Could you check a few things on this model? Use its own coordinates, in mm. A direction names the side the tool comes from. Coordinates: 2 decimals unless noted, no trailing zeros. Write each loop counter-clockwise with the first axis right and the second up, starting at its lowest first coordinate (ties: lowest second). Pieces come first, ordered by that corner, then holes.
Item 1: If I drill on probe 1 along Z at (x, y) = (-2.75, -4); probe 2 along X at (y, z) = (-1.25, 2.05); probe 3 along X at (y, z) = (5, 0.7), over which ranges is the centre line in solid material (lowest first)?
Item 2: I want a section at B-B on z = 2.8. Please give me the cut outline in (x, y), then the cut area to 3 significant figures.
Item 3: I want a section at A-A on z = 2. Please give me the cut outline in (x, y), then the cut area to 3 significant figures.
Item 4: For P1, Ø1, axis at x = -3.5, y = 5, coming from the +Z side, with a flat end and sliding along its axis, tell me the tip position at first contact or that it passes through.
Item 5: Which directions (+Z, -Z, +X, -X, +Y, -Y) give clear straight access to the entire face, cutting with the end or side of a thin tool? Please do faces 1 (the flat face through (0, 0, 3.2)), 2 (the flat face through (-5, 0, 3.12)).
Solid Edge part; units mm, degrees
sketch "Sketch1" plane through (0, 0, 0) normal (0, -1, 0) x (1, 0, 0)
  line L0 (0, 3.2) -> (4.2802, 3.2)
  line L1 (4.2802, 3.2) -> (4.5, 3.12)
  line L2 (4.5, 3.12) -> (6.25, 3.12)
  line L3 (6.25, 3.12) -> (6.25, 0)
  line L4 (6.25, 0) -> (0, 0)
  dimension "D1" = 6.25
  dimension "D2" = 4.2802
revolve "RevolvedProtrusion1" add sketch "Sketch1" angle 360 about axis through (0, 0, 0) along (0, 0, 1)
fillet "Round1" radius 0.75 2 edges at (-6.25, 0, 3.12) (-4.2802, 0, 3.2)
fillet "Round_2" radius 0.15 1 edges at (-6.25, 0, 0)
Response values:
1. probe 1: z = 0 to 3.12
1. probe 2: x = -6.12 to 6.12
1. probe 3: x = -3.75 to 3.75
2. outline: circle Ø12.23 at (0, 0)
2. area: 117 mm2
3. outline: circle Ø12.5 at (0, 0)
3. area: 123 mm2
4. P1: stops at z = 3.11
5. face 1: +Z, +X, -X, +Y, -Y
5. face 2: +Z
